Read the model definition and answer for the solid it produces. Units are mm, in the model's axes. A direction names the side the tool comes from. Round coordinates to 2 decimals unless told otherwise and drop trailing zeros. Write each loop counter-clockwise with the first axis right and the second up, starting at its lowest first coordinate (ties: lowest second). Pieces come first, ordered by that corner, then holes. Notation, with made-up numbers: (65.25, 86.25) -> (114.25, 86.25) arc R19 cw to (114.25, 94.25) -> close; hole circle Ø4 at (11.5, 30). An arc over 180 degrees is marked (long way). Return JSON: item names as keys, results as strings. Group by question number.
(1) For faces 1 (the flat face through (65, 0, 6)), 2 (the cylindrical face through (64.93, 5.314, -5.293)), 3 (the cylindrical face through (5.44, 1.73, -7.81)), 4 (the cylindrical face through (64.93, -5.314, 5.293)), 5 (the flat face through (60, -7, 0)), determine the directions among +Z, -Z, +X, -X, +Y, -Y from which every point of the face is accessible in a straight line to the end or side of a thin tool.
(2) Given pin 1 (4.5 mm diameter, centred on x = 67, y = -1, fed in from +Z); pin 2 (2 mm diameter, centred on y = -7.5, z = -3.5, fed in from +X); pin 3 (2 mm diameter, centred on x = 53.5, z = -7.5, fed in from -Y), each flat-ended and moving along its own axis, determine where each tip first touches the part or whether it passes through.
(3) A cutting plane is placed at D-D on x = 5.5. Give the vertices of the cut face in (y, z), then the cut area to 3 significant figures.
(4) A cutting plane is placed at C-C on x = 13.5. Give the vertices of the cut face in (y, z).
(5) Straight lines are drawn through the part: line 1 (X direction, y = -8, z = -2.75); line 2 (X direction, y = 6.25, z = 1); line 3 (Y direction, x = 16, z = 0.5). For each, find the intervals that lie inside material, in ascending order.
(6) A cutting plane is placed at A-A on z = 0. Give the vertices of the cut face in (x, y).
Autodesk Inventor part; units mm, degrees
ref_plane "YZ Plane" through (0, 0, 0) normal (1, 0, 0) x (0, 1, 0)
ref_plane "XZ Plane" through (0, 0, 0) normal (0, 1, 0) x (-1, 0, 0)
ref_plane "XY Plane" through (0, 0, 0) normal (0, 0, 1) x (1, 0, 0)
sketch "草图1" plane through (0, 0, 0) normal (0, 0, 1) x (1, 0, 0)
  line L0 (0, 0) -> (10, 0)
  line L1 (10, 0) -> (10, -8)
  line L2 (10, -8) -> (0, -8)
  line L3 (0, -8) -> (0, 0)
  line L4 (10, 0) -> (60, 0)
  line L5 (60, 0) -> (60, -12)
  line L6 (60, -12) -> (10, -12)
  line L7 (10, -12) -> (10, 0)
  dimension "d0" = 10
  dimension "d1" = 8
  dimension "d2" = 50
  dimension "d3" = 12
revolve "旋转1" add sketch "草图1" angle 360 about axis through (10, 0, 0) along (1, 0, 0)
chamfer "倒角1" distance 1 angle 45 1 edges at (60, 12, 0)
chamfer "倒角2" distance 1 angle 45 1 edges at (0, 8, 0)
chamfer "倒角3" distance 1 angle 45 1 edges at (10, 12, 0)
sketch "草图2" plane through (60, 0, 0) normal (1, 0, 0) x (0, 0, -1)
  line L0 (-4.5, 6) -> (4.5, 6)
  line L1 (6, 4.5) -> (6, -4.5)
  line L2 (4.5, -6) -> (-4.5, -6)
  line L3 (-6, -4.5) -> (-6, 4.5)
  line L4 (-6, 6) -> (6, -6) construction
  line L5 (6, 6) -> (-6, -6) construction
  arc A0 (-4.5, 6) -> (-6, 4.5) centre (0, 0) ccw
  arc A1 (-6, -4.5) -> (-4.5, -6) centre (0, 0) ccw
  arc A2 (4.5, -6) -> (6, -4.5) centre (0, 0) ccw
  arc A3 (6, 4.5) -> (4.5, 6) centre (0, 0) ccw
  dimension "d15" = 12
  dimension "d16" = 12
extrude "拉伸1" add sketch "草图2" along normal blind 10
thread "螺纹1"
properties part number "10-螺杆" material "不锈钢"
Checks:
{
 "1": {"face 1": "+Z, +X, +Y, -Y", "face 2": "-Z, +X, +Y", "face 3": "-X", "face 4": "+Z, +X, -Y", "face 5": "+X"},
 "2": {"pin 1": "stops at z = 6", "pin 2": "stops at x = 60", "pin 3": "stops at y = -10.09"},
 "3": {"outline": "circle Ø16 at (0, 0)", "area": "201 mm^2"},
 "4": {"outline": "circle Ø24 at (0, 0)"},
 "5": {"line 1": "x = 10 to 60", "line 2": "x = 0 to 60", "line 3": "y = -11.99 to 11.99"},
 "6": {"outline": "(0, -7) -> (1, -8) -> (10, -8) -> (10, -11) -> (11, -12) -> (59, -12) -> (60, -11) -> (60, -6) -> (70, -6) -> (70, 6) -> (60, 6) -> (60, 11) -> (59, 12) -> (11, 12) -> (10, 11) -> (10, 8) -> (1, 8) -> (0, 7) -> close"}
}
